from build123d import *

# Parameters (mm, degrees)
EXTRUDE_1_DEPTH      = 61
SKETCH_2_W           = 40
SKETCH_2_H           = 53
CUT_EXTRUDE_1_DEPTH  = 61
SKETCH_3_R           = 4
CUT_EXTRUDE_2_DEPTH  = 61
SKETCH_6_W           = 61
SKETCH_6_H           = 61
EXTRUDE_3_DEPTH      = 6
EXTRUDE_4_DEPTH      = 6
CUT_EXTRUDE_4_DEPTH  = 6
SKETCH_21_R          = 4
SKETCH_21_R_2        = 1.5
EXTRUDE_10_DEPTH     = 4
SKETCH_22_R          = 1.5
CUT_EXTRUDE_11_DEPTH = 4
SKETCH_23_W          = 61
SKETCH_23_H          = 61
CUT_EXTRUDE_12_DEPTH = 2
CUT_EXTRUDE_START    = -103
SKETCH_24_W          = 18.957699184
SKETCH_24_H          = 3.1
CUT_EXTRUDE_13_DEPTH = 141
SKETCH_25_R          = 4
SKETCH_25_R_2        = 1.5
EXTRUDE_11_DEPTH     = 4
SKETCH_26_R          = 1.5
EXTRUDE_12_DEPTH     = 7
CUT_EXTRUDE_14_DEPTH = 3
SKETCH_30_R          = 4.5
CUT_EXTRUDE_15_DEPTH = 46
EXTRUDE_14_DEPTH     = 0.6
EXTRUDE_15_DEPTH     = 0.6
EXTRUDE_16_DEPTH     = 1
EXTRUDE_16_TAPER     = 48
CUT_EXTRUDE_16_DEPTH = 1
CUT_EXTRUDE_17_DEPTH = 1


with BuildPart() as part:
    # 草图1 → 凸台-拉伸1 (new body)
    with BuildSketch(Plane(origin=(0, 0, 0), x_dir=(1, 0, 0), z_dir=(0, 1, 0))):
        with BuildLine():
            Line((43.616831607, -30.5), (50.616831607, -30.5))
            Line((50.616831607, -30.5), (50.616831607, 30.5))
            Line((50.616831607, 30.5), (43.616831607, 30.5))
            ThreePointArc((43.616831607, 30.5), (13.116831607, 0), (43.616831607, -30.5))
        make_face()
    extrude(amount=EXTRUDE_1_DEPTH)

    # 草图2 → 切除-拉伸1 (cut)
    with BuildSketch(Plane.XY.offset(30.5)):
        with Locations((26.616831607, 30.5)):
            Rectangle(SKETCH_2_W, SKETCH_2_H)
    extrude(amount=-CUT_EXTRUDE_1_DEPTH, mode=Mode.SUBTRACT)

    # 草图3 → 切除-拉伸2 (cut)
    with BuildSketch(Plane(origin=(0, 61, 0), x_dir=(1, 0, 0), z_dir=(0, 1, 0))):
        with Locations((24.116831607, 0)):
            Circle(SKETCH_3_R)
    extrude(amount=-CUT_EXTRUDE_2_DEPTH, mode=Mode.SUBTRACT)

    # 草图6 → 凸台-拉伸3 (add)
    with BuildSketch(Plane.ZY.offset(-46.616831607)):
        with Locations((0, 30.5)):
            Rectangle(SKETCH_6_W, SKETCH_6_H)
    extrude(amount=EXTRUDE_3_DEPTH)

    # 草图7 → 凸台-拉伸4 (add)
    with BuildSketch(Plane.XZ.offset(-57)):
        with BuildLine():
            Line((40.616831607, 30.352100422), (40.616831607, -30.352100422))
            ThreePointArc((40.616831607, -30.352100422), (13.116831607, 0), (40.616831607, 30.352100422))
        make_face()
    extrude_4 = extrude(amount=EXTRUDE_4_DEPTH)

    # 草图8 → 切除-拉伸4 (cut)
    with BuildSketch(Plane.XZ.offset(-51)):
        Polygon((9.690406562, -10), (9.690406562, 10), (24.116831607, 30.269119374), (34.616831607, 33.638775852), (34.616831607, -30.352100422), (24.116831607, -25.227142121), align=None)
    cut_extrude_4 = extrude(amount=-CUT_EXTRUDE_4_DEPTH, mode=Mode.SUBTRACT)

    # 草图21 → 凸台-拉伸10 (add)
    with BuildSketch(Plane(origin=(0, 61, 0), x_dir=(1, 0, 0), z_dir=(0, 1, 0))):
        with Locations((24.116831607, 0)):
            Circle(SKETCH_21_R)
        with Locations((24.116831607, 0)):
            Circle(SKETCH_21_R_2, mode=Mode.SUBTRACT)
    extrude(amount=-EXTRUDE_10_DEPTH)

    # 草图22 → 切除-拉伸11 (cut)
    with BuildSketch(Plane(origin=(0, 61, 0), x_dir=(1, 0, 0), z_dir=(0, 1, 0))):
        with Locations((31.116831607, 0)):
            Circle(SKETCH_22_R)
        with Locations((24.116831607, -7)):
            Circle(SKETCH_22_R)
        with Locations((17.116831607, 0)):
            Circle(SKETCH_22_R)
        with Locations((24.116831607, 7)):
            Circle(SKETCH_22_R)
    cut_extrude_11 = extrude(amount=-CUT_EXTRUDE_11_DEPTH, mode=Mode.SUBTRACT)

    # 草图23 → 切除-拉伸12 (cut)
    with BuildSketch(Plane(origin=(50.616831607, 0, 0), x_dir=(0, 0, -1), z_dir=(1, 0, 0))):
        with Locations((0, 30.5)):
            Rectangle(SKETCH_23_W, SKETCH_23_H)
    extrude(amount=-CUT_EXTRUDE_12_DEPTH, mode=Mode.SUBTRACT)

    # 草图24 → 切除-拉伸13 (cut)
    with BuildSketch(Plane.XY.offset(30.5).offset(CUT_EXTRUDE_START)):
        with Locations((31.137982015, 52.55)):
            Rectangle(SKETCH_24_W, SKETCH_24_H)
    cut_extrude_13 = extrude(amount=CUT_EXTRUDE_13_DEPTH, mode=Mode.SUBTRACT)

    # 镜向1: 凸台-拉伸4, 切除-拉伸4, 切除-拉伸11, 切除-拉伸13 across plane
    add(extrude_4.mirror(Plane(origin=(0, 30.5, 0), x_dir=(0, 0, 1), z_dir=(0, -1, 0))))
    add(cut_extrude_4.mirror(Plane(origin=(0, 30.5, 0), x_dir=(0, 0, 1), z_dir=(0, -1, 0))), mode=Mode.SUBTRACT)
    add(cut_extrude_11.mirror(Plane(origin=(0, 30.5, 0), x_dir=(0, 0, 1), z_dir=(0, -1, 0))), mode=Mode.SUBTRACT)
    add(cut_extrude_13.mirror(Plane(origin=(0, 30.5, 0), x_dir=(0, 0, 1), z_dir=(0, -1, 0))), mode=Mode.SUBTRACT)

    # 草图25 → 凸台-拉伸11 (add)
    with BuildSketch(Plane.XZ):
        with Locations((24.116831607, 0)):
            Circle(SKETCH_25_R)
        with Locations((24.116831607, 0)):
            Circle(SKETCH_25_R_2, mode=Mode.SUBTRACT)
    extrude(amount=-EXTRUDE_11_DEPTH)

    # 草图26 → 凸台-拉伸12 (add)
    with BuildSketch(Plane.XY.offset(30.5)):
        Polygon((48.616831607, 12.5), (48.616831607, 48.5), (78.616831607, 41.256266774), (78.616831607, 19.743733226), align=None)
        with Locations((65.616831607, 30.5)):
            Circle(SKETCH_26_R, mode=Mode.SUBTRACT)
        with Locations((65.616831607, 37.5)):
            Circle(SKETCH_26_R, mode=Mode.SUBTRACT)
        with Locations((72.616831607, 30.5)):
            Circle(SKETCH_26_R, mode=Mode.SUBTRACT)
        with Locations((65.616831607, 23.5)):
            Circle(SKETCH_26_R, mode=Mode.SUBTRACT)
        with Locations((58.616831607, 30.5)):
            Circle(SKETCH_26_R, mode=Mode.SUBTRACT)
    extrude_12 = extrude(amount=-EXTRUDE_12_DEPTH)

    # 草图27 → 切除-拉伸14 (cut)
    with BuildSketch(Plane(origin=(0, 0, 23.5), x_dir=(-1, 0, 0), z_dir=(0, 0, -1))):
        Polygon((-65.616831607, 49.155948688), (-88.62878141, 40.6), (-88.62878141, 5.471682321), (-65.616831607, 5.471682321), (-55.516831607, 5.471682321), (-54.616831607, 7.907008969), (-54.616831607, 48.5), (-55.516831607, 53.096755827), align=None)
    cut_extrude_14 = extrude(amount=-CUT_EXTRUDE_14_DEPTH, mode=Mode.SUBTRACT)

    # 镜向2: 凸台-拉伸12, 切除-拉伸14 across plane
    add(extrude_12.mirror(Plane.XY))
    add(cut_extrude_14.mirror(Plane.XY), mode=Mode.SUBTRACT)

    # 草图30 → 切除-拉伸15 (cut)
    with BuildSketch(Plane(origin=(48.616831607, 0, 0), x_dir=(0, 0, -1), z_dir=(1, 0, 0))):
        with Locations((-15.25, 30.5)):
            Circle(SKETCH_30_R)
        with Locations((15.25, 30.5)):
            Circle(SKETCH_30_R)
    extrude(amount=-CUT_EXTRUDE_15_DEPTH, mode=Mode.SUBTRACT)

    # 草图31 → 凸台-拉伸14 (add)
    with BuildSketch(Plane(origin=(0, 61, 0), x_dir=(1, 0, 0), z_dir=(0, 1, 0))):
        Polygon((48.616831607, 30.5), (34.786624989, 0), (48.616831607, -30.5), align=None)
    extrude_14 = extrude(amount=EXTRUDE_14_DEPTH)

    # 草图32 → 凸台-拉伸15 (add)
    with BuildSketch(Plane(origin=(0, 61.6, 0), x_dir=(1, 0, 0), z_dir=(0, 1, 0))):
        Polygon((48.616831607, 23.5), (37.328660261, 0), (48.616831607, -23.5), align=None)
    extrude_15 = extrude(amount=EXTRUDE_15_DEPTH)

    # 草图33 → 凸台-拉伸16 (add)
    with BuildSketch(Plane(origin=(0, 62.2, 0), x_dir=(1, 0, 0), z_dir=(0, 1, 0))):
        Polygon((48.616831607, 18.308068361), (40.592556225, 0), (48.616831607, -18.308068361), align=None)
    extrude_16 = extrude(amount=EXTRUDE_16_DEPTH, taper=EXTRUDE_16_TAPER)

    # 草图34 → 切除-拉伸16 (cut)
    with BuildSketch(Plane(origin=(0, 61, 0), x_dir=(1, 0, 0), z_dir=(0, 1, 0))):
        Polygon((36.215945499, 9.330034221), (48.049296547, 32.77894458), (47.156533889, 33.229471866), (35.271831325, 9.678803595), align=None)
        Polygon((27.787246694, 12.443716957), (26.84313252, 12.792486331), (37.156533889, 33.229471866), (38.049296547, 32.77894458), align=None)
        Polygon((32.001596097, 10.886875589), (43.049296547, 32.77894458), (42.156533889, 33.229471866), (31.057481922, 11.235644963), align=None)
        Polygon((23.572897292, 14.000558325), (22.628783117, 14.349327699), (32.156533889, 33.229471866), (33.049296547, 32.77894458), align=None)
        Polygon((32.001596097, -10.886875589), (31.057481922, -11.235644963), (42.156533889, -33.229471866), (43.049296547, -32.77894458), align=None)
        Polygon((36.215945499, -9.330034221), (35.271831325, -9.678803595), (47.156533889, -33.229471866), (48.049296547, -32.77894458), align=None)
        Polygon((33.049296547, -32.77894458), (32.156533889, -33.229471866), (22.628783117, -14.349327699), (23.572897292, -14.000558325), align=None)
        Polygon((38.049296547, -32.77894458), (37.156533889, -33.229471866), (26.84313252, -12.792486331), (27.787246694, -12.443716957), align=None)
    cut_extrude_16 = extrude(amount=-CUT_EXTRUDE_16_DEPTH, mode=Mode.SUBTRACT)

    # 草图35 → 切除-拉伸17 (cut)
    with BuildSketch(Plane.XY.offset(30.5)):
        Polygon((50.215248512, 44.601766544), (43.170813126, 31.382579155), (53.95488705, 31.382579155), (46.430297324, 17.262361399), (58.129367278, 34.600407664), (47.258325017, 33.382850931), align=None)
    cut_extrude_17 = extrude(amount=-CUT_EXTRUDE_17_DEPTH, mode=Mode.SUBTRACT)

    # 镜向3: 切除-拉伸17 across plane
    add(cut_extrude_17.mirror(Plane.XY), mode=Mode.SUBTRACT)

    # 镜向4: 凸台-拉伸14, 凸台-拉伸15, 凸台-拉伸16, 切除-拉伸16 across plane
    add(extrude_14.mirror(Plane(origin=(0, 30.5, 0), x_dir=(0, 0, 1), z_dir=(0, -1, 0))))
    add(extrude_15.mirror(Plane(origin=(0, 30.5, 0), x_dir=(0, 0, 1), z_dir=(0, -1, 0))))
    add(extrude_16.mirror(Plane(origin=(0, 30.5, 0), x_dir=(0, 0, 1), z_dir=(0, -1, 0))))
    add(cut_extrude_16.mirror(Plane(origin=(0, 30.5, 0), x_dir=(0, 0, 1), z_dir=(0, -1, 0))), mode=Mode.SUBTRACT)


solid = part.part
Model file for the job. Use its own axes, mm. A direction names the side the tool comes from. Give positions to 0.01 mm unless a question says otherwise; leave off trailing zeros. Order: outer loops, then holes, each group sorted by start corner. A loop starts at its lowest first (then second) coordinate and runs counter-clockwise, first axis right, second up. Notation, with made-up numbers: (-6, 40) -> (44, 40) arc R11 cw to (44, 58) -> close; hole circle Ø9 at (70, 0.5). An arc over 180 degrees is marked (long way). Use CSV: the item, a comma, the result in double quotes.
1. Band-saw the part on B-B, the plane x = 72.5. Give the cut face in (y, z).
Outcome:
outline,"(18.27, -30.5) -> (29, -30.5) -> (29, -26.5) -> (18.27, -26.5) -> close; (18.27, 26.5) -> (29, 26.5) -> (29, 30.5) -> (18.27, 30.5) -> close; (32, -30.5) -> (42.73, -30.5) -> (42.73, -26.5) -> (32, -26.5) -> close; (32, 26.5) -> (42.73, 26.5) -> (42.73, 30.5) -> (32, 30.5) -> close"
2. Band-saw the part on A-A, the plane y = 23.5. Give the cut face in (x, z).
Outcome:
outline,"(40.62, -30.5) -> (49.75, -30.5) -> (49.75, -29.5) -> (50.64, -29.5) -> (50.64, -30.5) -> (64.12, -30.5) -> (64.12, -26.5) -> (54.62, -26.5) -> (54.62, -23.5) -> (48.62, -23.5) -> (48.62, 23.5) -> (54.62, 23.5) -> (54.62, 26.5) -> (64.12, 26.5) -> (64.12, 30.5) -> (50.64, 30.5) -> (50.64, 29.5) -> (49.75, 29.5) -> (49.75, 30.5) -> (40.62, 30.5) -> close; (67.12, -30.5) -> (78.62, -30.5) -> (78.62, -26.5) -> (67.12, -26.5) -> close; (67.12, 26.5) -> (78.62, 26.5) -> (78.62, 30.5) -> (67.12, 30.5) -> close"
3. Mould opens along X. For faces 1 (the flat face through (38, 54.1, 0)), 2 (the flat face through (54.617, 30, -25)), 3 (the flat face through (26.925, 60.507, 20.643)) say: +X half, -X half, draft (parallel to the pull), parting line (faces both ways), or undercut.
Outcome:
face 1,"draft"
face 2,"+X half"
face 3,"undercut"
4. Drill centre lines: line 1 along X through (y, z) = (1.4, -7); line 2 along Z through (x, y) = (48.5, 32); line 3 along X through (y, z) = (46, -7). Where is each one in solid material? Low to high. Write a range as from..to.
Outcome:
line 1,"13.93..22.62, 25.62..48.62"
line 2,"-29.5..-19.49, -11.01..11.01, 19.49..29.5"
line 3,"40.62..48.62"
5. 3-axis set-ups, long thin cutter, end or side, ignore diameter. For faces 4 (the flat face through (32.19, 0.49, -21.17)), 5 (the flat face through (36.5, 60, 20.6)), 6 (the cylindrical face through (66.31, 36.17, -28.53)): which of +Z, -Z, +X, -X, +Y, -Y reach the whole face in a straight line?
Outcome:
face 4,"-Y"
face 5,"+Y"
face 6,"+Z, -Z"
6. Band-saw the part on C-C, the plane y = 37.5. Give the cut face in (x, z), then the cut area to 3 significant figures.
Outcome:
outline,"(40.62, -30.5) -> (46.43, -30.5) -> (46.43, -29.5) -> (48.34, -29.5) -> (48.34, -30.5) -> (64.12, -30.5) -> (64.12, -26.5) -> (54.62, -26.5) -> (54.62, -23.5) -> (48.62, -23.5) -> (48.62, 23.5) -> (54.62, 23.5) -> (54.62, 26.5) -> (64.12, 26.5) -> (64.12, 30.5) -> (48.34, 30.5) -> (48.34, 29.5) -> (46.43, 29.5) -> (46.43, 30.5) -> (40.62, 30.5) -> close; (67.12, -30.5) -> (78.62, -30.5) -> (78.62, -26.5) -> (67.12, -26.5) -> close; (67.12, 26.5) -> (78.62, 26.5) -> (78.62, 30.5) -> (67.12, 30.5) -> close"
area,"736 mm²"
7. Band-saw the part on D-D, the plane z = 7. Count the separate pieces of the cut face and the enclosed holes in it, then the cut area to 3 significant figures.
Outcome:
separate pieces,"3"
enclosed holes,"0"
area,"742 mm²"
8. Drop flat-ended pins along their axis: pin 1 (4 mm diameter, centred on x = 31.12, z = 0, fed in from -Y); pin 2 (1.5 mm diameter, centred on y = 29.5, z = -22.5, fed in from -X); pin 3 (5 mm diameter, centred on x = 17.12, z = 0, fed in from +Y); pin 4 (7 mm diameter, centred on y = 30.5, z = 15.25, fed in from -X). Give the stop position or say it passes through.
Outcome:
pin 1,"y = 0"
pin 2,"x = 40.62"
pin 3,"y = 61"
pin 4,"through"
